Source: CAD feature listing. Evaluate the final solid. Frame: model axes, mm. Face numbers are marked on the shaded views. A direction names the side the tool comes from. Give positions to 0.01 mm unless a question says otherwise; leave off trailing zeros. Loops run counter-clockwise (first coordinate to the right, second up) from the corner with the lowest first, then second, coordinate; pieces in that order, holes last. Notation, with made-up numbers: M 52.25,-30.5 L 90.25,-30.5 A25 ccw 90.25,-11.5 Z; hole C 16,50 d8. An arc over 180 degrees is marked long. Write item = value, one per line.
from build123d import *

# Parameters (mm, degrees)
BOSS_EXTRUDE1_DEPTH = 10.5
SKETCH2_R           = 1.5
CUT_EXTRUDE1_DEPTH  = 10.5


with BuildPart() as part:
    # Sketch1 → Boss-Extrude1 (new body)
    with BuildSketch(Plane(origin=(0, 0, 0), x_dir=(1, 0, 0), z_dir=(0, 1, 0))):
        with BuildLine():
            ThreePointArc((1.04, 5.400777722), (0.783531714, 6.485041414), (0.31, 7.493590595))
            ThreePointArc((0.31, 7.493590595), (0, 7.5), (-0.31, 7.493590595))
            ThreePointArc((-0.31, 7.493590595), (-0.783531714, 6.485041414), (-1.04, 5.400777722))
            ThreePointArc((-1.04, 5.400777722), (-1.316236154, 5.340179996), (-1.588992288, 5.265463276))
            ThreePointArc((-1.588992288, 5.265463276), (-2.319966139, 6.10634434), (-3.207953823, 6.779309129))
            ThreePointArc((-3.207953823, 6.779309129), (-3.48542379, 6.640920192), (-3.756936559, 6.491180762))
            ThreePointArc((-3.756936559, 6.491180762), (-3.707531894, 5.378093653), (-3.430740821, 4.298839078))
            ThreePointArc((-3.430740821, 4.298839078), (-3.64717462, 4.116809115), (-3.853965592, 3.923894649))
            ThreePointArc((-3.853965592, 3.923894649), (-4.891987708, 4.328757368), (-5.991004086, 4.511969642))
            ThreePointArc((-5.991004086, 4.511969642), (-6.172378994, 4.2604856), (-6.343204228, 4.001719645))
            ThreePointArc((-6.343204228, 4.001719645), (-5.782181198, 3.039089449), (-5.035540265, 2.212088208))
            ThreePointArc((-5.035540265, 2.212088208), (-5.142589335, 1.950326879), (-5.236041824, 1.683409046))
            ThreePointArc((-5.236041824, 1.683409046), (-6.343313848, 1.559504249), (-7.401587511, 1.210992284))
            ThreePointArc((-7.401587511, 1.210992284), (-7.445316556, 0.904025102), (-7.476320253, 0.595512782))
            ThreePointArc((-7.476320253, 0.595512782), (-6.532202472, 0.003866477), (-5.486758119, -0.381425412))
            ThreePointArc((-5.486758119, -0.381425412), (-5.459898808, -0.662951741), (-5.418603976, -0.942725282))
            ThreePointArc((-5.418603976, -0.942725282), (-6.341463231, -1.567012498), (-7.116556437, -2.367408811))
            ThreePointArc((-7.116556437, -2.367408811), (-7.01262182, -2.659536653), (-6.896701407, -2.947118882))
            ThreePointArc((-6.896701407, -2.947118882), (-5.785774881, -3.032242258), (-4.68102581, -2.887559066))
            ThreePointArc((-4.68102581, -2.887559066), (-4.526411262, -3.124356107), (-4.359829258, -3.352892609))
            ThreePointArc((-4.359829258, -3.352892609), (-4.886859811, -4.334545567), (-5.201208047, -5.403465078))
            ThreePointArc((-5.201208047, -5.403465078), (-4.973419937, -5.613830611), (-4.737131383, -5.814601127))
            ThreePointArc((-4.737131383, -5.814601127), (-3.713895991, -5.373700834), (-2.802926901, -4.732187738))
            ThreePointArc((-2.802926901, -4.732187738), (-2.555977446, -4.870008141), (-2.302270198, -4.994952646))
            ThreePointArc((-2.302270198, -4.994952646), (-2.312735701, -6.109086484), (-2.094325574, -7.201652615))
            ThreePointArc((-2.094325574, -7.201652615), (-1.794867482, -7.282063631), (-1.492341648, -7.350028327))
            ThreePointArc((-1.492341648, -7.350028327), (-0.791208287, -6.484109309), (-0.282711218, -5.492729228))
            ThreePointArc((-0.282711218, -5.492729228), (0, -5.5), (0.282711218, -5.492729228))
            ThreePointArc((0.282711218, -5.492729228), (0.791208287, -6.484109309), (1.492341648, -7.350028327))
            ThreePointArc((1.492341648, -7.350028327), (1.794867482, -7.282063631), (2.094325574, -7.201652615))
            ThreePointArc((2.094325574, -7.201652615), (2.312735701, -6.109086484), (2.302270198, -4.994952646))
            ThreePointArc((2.302270198, -4.994952646), (2.555977446, -4.870008141), (2.802926901, -4.732187738))
            ThreePointArc((2.802926901, -4.732187738), (3.713895991, -5.373700834), (4.737131383, -5.814601127))
            ThreePointArc((4.737131383, -5.814601127), (4.973419937, -5.613830611), (5.201208047, -5.403465078))
            ThreePointArc((5.201208047, -5.403465078), (4.886859811, -4.334545567), (4.359829258, -3.352892609))
            ThreePointArc((4.359829258, -3.352892609), (4.526411262, -3.124356107), (4.68102581, -2.887559066))
            ThreePointArc((4.68102581, -2.887559066), (5.785774881, -3.032242258), (6.896701407, -2.947118882))
            ThreePointArc((6.896701407, -2.947118882), (7.01262182, -2.659536653), (7.116556437, -2.367408811))
            ThreePointArc((7.116556437, -2.367408811), (6.341463231, -1.567012498), (5.418603976, -0.942725282))
            ThreePointArc((5.418603976, -0.942725282), (5.459898808, -0.662951741), (5.486758119, -0.381425412))
            ThreePointArc((5.486758119, -0.381425412), (6.532202472, 0.003866477), (7.476320253, 0.595512782))
            ThreePointArc((7.476320253, 0.595512782), (7.445316556, 0.904025102), (7.401587511, 1.210992284))
            ThreePointArc((7.401587511, 1.210992284), (6.343313848, 1.559504249), (5.236041824, 1.683409046))
            ThreePointArc((5.236041824, 1.683409046), (5.142589335, 1.950326879), (5.035540265, 2.212088208))
            ThreePointArc((5.035540265, 2.212088208), (5.782181198, 3.039089449), (6.343204228, 4.001719645))
            ThreePointArc((6.343204228, 4.001719645), (6.172378994, 4.2604856), (5.991004086, 4.511969642))
            ThreePointArc((5.991004086, 4.511969642), (4.891987708, 4.328757368), (3.853965592, 3.923894649))
            ThreePointArc((3.853965592, 3.923894649), (3.64717462, 4.116809115), (3.430740821, 4.298839078))
            ThreePointArc((3.430740821, 4.298839078), (3.707531894, 5.378093653), (3.756936559, 6.491180762))
            ThreePointArc((3.756936559, 6.491180762), (3.48542379, 6.640920192), (3.207953823, 6.779309129))
            ThreePointArc((3.207953823, 6.779309129), (2.319966139, 6.10634434), (1.588992288, 5.265463276))
            ThreePointArc((1.588992288, 5.265463276), (1.316236154, 5.340179996), (1.04, 5.400777722))
        make_face()
    extrude(amount=BOSS_EXTRUDE1_DEPTH)

    # Sketch2 → Cut-Extrude1 (cut)
    with BuildSketch(Plane(origin=(0, 10.5, 0), x_dir=(1, 0, 0), z_dir=(0, 1, 0))):
        Circle(SKETCH2_R)
    extrude(amount=-CUT_EXTRUDE1_DEPTH, mode=Mode.SUBTRACT)


solid = part.part
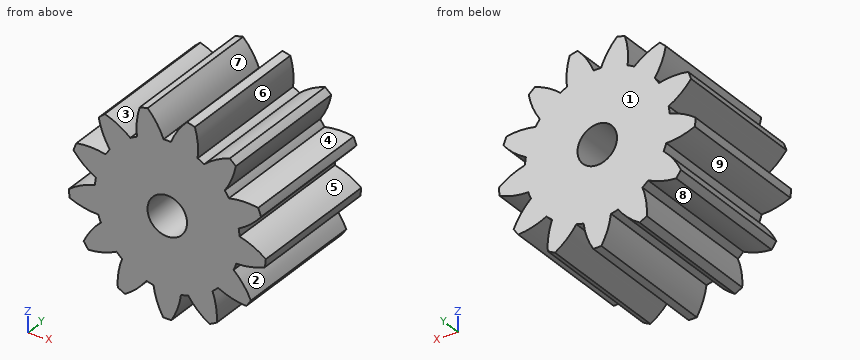
1. Cut plane D-D, the plane x = -3. Return the cut outline in (y, z).
Derived:
outline = M 0,-6.65 L 10.5,-6.65 L 10.5,4.9 L 0,4.9 Z
2. First-contact query: pin 1 Ø5 at (x, y) = (-2, 5.5) entering from +Z; pin 2 Ø4 at (x, y) = (5.5, 4) entering from +Z. Flat tips, straight axial feed; report the tip coordinate or a pass-through.
Derived:
pin_1 = 7.35
pin_2 = 5.81
3. Cut plane C-C, the plane z = -3. Return the cut outline in (x, y).
Derived:
outline = M -5.75,0 L 5.75,0 L 5.75,10.5 L -5.75,10.5 Z
4. Pull-direction query (X, two-part tool) for the marked faces 1, 2, 3 and 4; classes: +X half, -X half, draft (parallel to the pull), parting line (faces both ways), or undercut.
Derived:
face_1 = draft
face_2 = +X half
face_3 = undercut
face_4 = undercut
5. Cut plane B-B, the plane z = 6.5. Return the cut outline in (x, y).
Derived:
outline = M -2.26,0 L -0.8,0 L -0.8,10.5 L -2.26,10.5 Z; M 0.8,0 L 2.26,0 L 2.26,10.5 L 0.8,10.5 Z
6. Material intervals for probe 1 along X at (y, z) = (8.75, -6); probe 2 along X at (y, z) = (7.5, 0.75); probe 3 along X at (y, z) = (5.75, 0), sorted ascending. Write a range as from..to.
Derived:
probe_1 = -3.76..-2.21, -0.93..0.93, 2.21..3.76
probe_2 = -5.45..-1.3, 1.3..5.45
probe_3 = -6.52..-1.5, 1.5..6.52
7. Reachability of the marked faces 5, 6, 7, 8 and 9 from +Z, -Z, +X, -X, +Y, -Y: full face, straight path, thin tool, end or side. Return the list, or none.
Derived:
face_5 = +X, +Y, -Y
face_6 = +Y, -Y
face_7 = +Z, +Y, -Y
face_8 = -Z, +Y, -Y
face_9 = -X, +Y, -Y
8. Cut plane A-A, the plane x = 0. Return the cut outline in (y, z), then the cut area to 3 significant figures.
Derived:
outline = M 0,-7.5 L 10.5,-7.5 L 10.5,-1.5 L 0,-1.5 Z; M 0,1.5 L 10.5,1.5 L 10.5,5.5 L 0,5.5 Z
area = 105 mm²
